Autodesk Inventor part; units mm, degrees
ref_plane "YZ Plane" through (0, 0, 0) normal (1, 0, 0) x (0, 1, 0)
ref_plane "XZ Plane" through (0, 0, 0) normal (0, 1, 0) x (-1, 0, 0)
ref_plane "XY Plane" through (0, 0, 0) normal (0, 0, 1) x (1, 0, 0)
sketch "Sketch1" plane through (0, 0, 0) normal (0, 1, 0) x (-1, 0, 0)
  line L0 (0, 0) -> (25, 0)
  line L1 (25, 0) -> (25, -140)
  line L2 (25, -140) -> (0, -140)
  line L3 (0, -140) -> (0, 0)
  circle A0 centre (12.5, -10) radius 3.05
  circle A1 centre (12.5, -70) radius 3.05
  circle A2 centre (12.5, -130) radius 3.05
  line L4 (25, -70) -> (0, -70) construction
  line L5 (12.5, 0) -> (12.5, -140) construction
  circle A3 centre (12.5, -40) radius 3.05
  circle A4 centre (12.5, -100) radius 3.05
  dimension "d0" = 25
  dimension "d1" = 140
  dimension "d2" = 6.1
  dimension "d3" = 6.1
  dimension "d4" = 6.1
  dimension "d5" = 10
  dimension "d6" = 10
  dimension "d7" = 6.1
  dimension "d8" = 6.1
  dimension "d9" = 30
  dimension "d10" = 30
extrude "Extrusion1" add sketch "Sketch1" along normal blind 2.5
fillet "Fillet1" radius 2 4 edges at (0, 1.25, 0) (-25, 1.25, 0) (0, 1.25, -140) (-25, 1.25, -140)
equation "\"BendRadius\" = Thickness"
equation "\"BendReliefWidth\" = Thickness"
equation "\"BendReliefDepth\" = 0.5 * Thickness"
equation "\"CornerReliefSize\" = 4 * Thickness"
equation "\"MinimumRemnant\" = 2 * Thickness"
equation "\"TransitionRadius\" = BendRadius"
equation "\"JacobiRadiusSize\" = BendRadius"
equation "\"GapSize\" = Thickness"
properties part number "Connector"
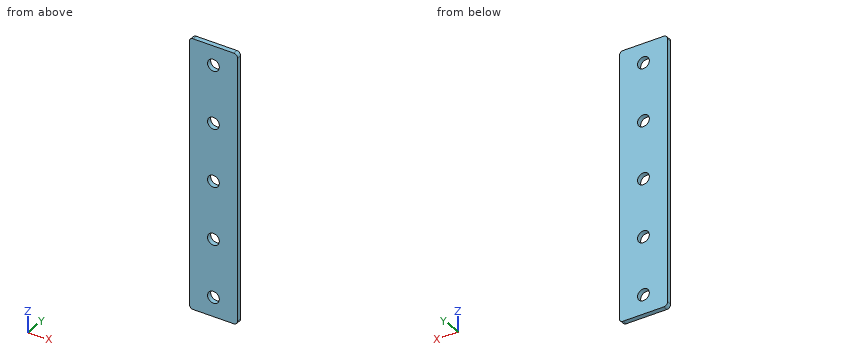
The model under review builds one solid part; all positions refer to its coordinate system, in mm. Round coordinates to 2 decimals unless told otherwise and drop trailing zeros. Loops run counter-clockwise (first coordinate to the right, second up) from the corner with the lowest first, then second, coordinate; pieces in that order, holes last. Notation, with made-up numbers: (14.5, 39) -> (65.5, 39) arc R17 ccw to (65.5, 68) -> close; hole circle Ø11 at (0.5, 55). An arc over 180 degrees is marked (long way). Answer as CSV lines item,"result".
1) Add section B-B on x = -12.5. Write out the cut boundary in (y, z).
Geometry results:
outline,"(0, -140) -> (2.5, -140) -> (2.5, -133.05) -> (0, -133.05) -> close; (0, -126.95) -> (2.5, -126.95) -> (2.5, -103.05) -> (0, -103.05) -> close; (0, -96.95) -> (2.5, -96.95) -> (2.5, -73.05) -> (0, -73.05) -> close; (0, -66.95) -> (2.5, -66.95) -> (2.5, -43.05) -> (0, -43.05) -> close; (0, -36.95) -> (2.5, -36.95) -> (2.5, -13.05) -> (0, -13.05) -> close; (0, -6.95) -> (2.5, -6.95) -> (2.5, 0) -> (0, 0) -> close"
2) Add section A-A on z = -40. Write out the cut boundary in (x, y), plus the area to 4 significant figures.
Geometry results:
outline,"(-25, 0) -> (-15.55, 0) -> (-15.55, 2.5) -> (-25, 2.5) -> close; (-9.45, 0) -> (0, 0) -> (0, 2.5) -> (-9.45, 2.5) -> close"
area,"47.25 mm²"
3) Add section C-C on y = 1.4. Write out the cut boundary in (x, z), plus the area to 3 significant figures.
Geometry results:
outline,"(-25, -138) arc R2 ccw to (-23, -140) -> (-2, -140) arc R2 ccw to (0, -138) -> (0, -2) arc R2 ccw to (-2, 0) -> (-23, 0) arc R2 ccw to (-25, -2) -> close; hole circle Ø6.1 at (-12.5, -130); hole circle Ø6.1 at (-12.5, -100); hole circle Ø6.1 at (-12.5, -70); hole circle Ø6.1 at (-12.5, -40); hole circle Ø6.1 at (-12.5, -10)"
area,"3,350 mm²"
4) To check wall thickness, follow line 1 along Z through (x, y) = (-12.5, 0.95); line 2 along Z through (x, y) = (-14, 0.7); line 3 along X through (y, z) = (1.3, -130). State the ranges of each line that lie inside material, in increasing order. Write a range as from..to.
Geometry results:
line 1,"z = -140..-133.05, -126.95..-103.05, -96.95..-73.05, -66.95..-43.05, -36.95..-13.05, -6.95..0"
line 2,"z = -140..-132.66, -127.34..-102.66, -97.34..-72.66, -67.34..-42.66, -37.34..-12.66, -7.34..0"
line 3,"x = -25..-15.55, -9.45..0"
5) For P1, Ø3.5, axis at x = -12.5, z = -130, coming from the -Y side, flat-tipped, find the tip position at first contact; note if it passes through.
Geometry results:
P1,"passes through"
